Input: dimensioned drawing with shaded views. Units: mm. Origin: part minimum x, y, z. A direction names the side the tool comes from. Coordinates: 2 decimals unless noted, no trailing zeros. Order: outer loops, then holes, each group sorted by start corner. A loop starts at its lowest first (then second) coordinate and runs counter-clockwise, first axis right, second up. Notation, with made-up numbers: (71.25, 5.25) -> (112.25, 5.25) arc R22 cw to (112.25, 20.25) -> close; hole circle Ø11 at (72, 5.25). An arc over 180 degrees is marked (long way). Answer in a Markdown table with one row per item. Add a question column.
1) Pull-direction query (Z, two-part tool) for the marked faces 1, 2 and 3; classes: +Z half, -Z half, draft (parallel to the pull), parting line (faces both ways), or undercut.
2) Section query A-A on z = 0.4. Return the cut outline in (x, y), then the cut area to 3 significant figures.
3) Ray query, line 1 (Y direction, x = 20.82, z = 1.6); line 2 (X direction, y = 11, z = 1.75); line 3 (Y direction, x = 19.25, z = 2.75). Return the intervals inside material, ascending. Write a range as from..to.
4) Set-up query: the marked faces 4 and 5. Return all of +Z, -Z, +X, -X, +Y, -Y with unobstructed straight access to the full face (end or side cutting, diameter ignored); none if empty.
5) Section query C-C on y = 7.9. Return the cut outline in (x, z) (1 decimal).
6) Contact query for flat-ended pins moving along their axis: P1, Ø1, axis at x = 11, z = 1, coming from the -Y side; P2, Ø3.5, axis at x = 8.82, y = 34, coming from the +Z side (1 decimal). Output: stop coordinate, or through.
7) Section query D-D on y = 34. Return the cut outline in (x, z) (1 decimal).
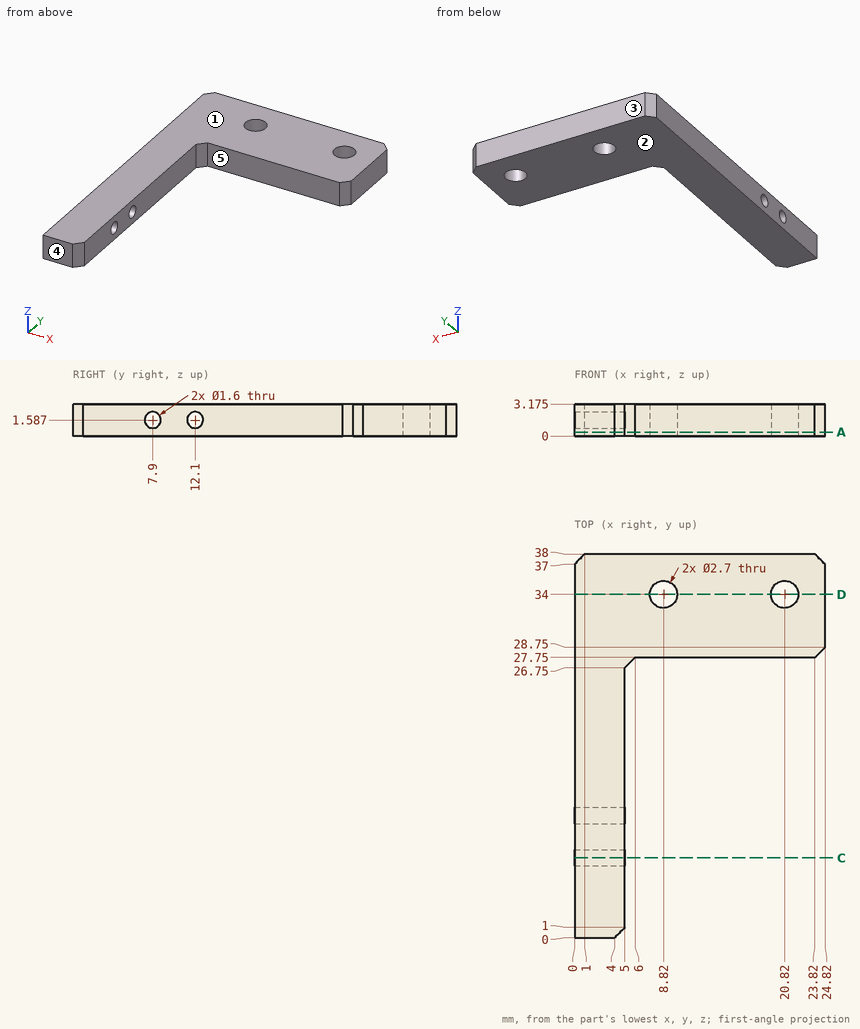
Result:
| question | item | result |
|---|---|---|
| 1 | face 1 | +Z half |
| 1 | face 2 | -Z half |
| 1 | face 3 | draft |
| 2 | outline | (0, 0) -> (4, 0) -> (5, 1) -> (5, 26.75) -> (6, 27.75) -> (23.82, 27.75) -> (24.82, 28.75) -> (24.82, 37) -> (23.82, 38) -> (1, 38) -> (0, 37) -> close; hole circle Ø2.7 at (8.82, 34); hole circle Ø2.7 at (20.82, 34) |
| 2 | area | 380 mm2 |
| 3 | line 1 | 27.75..32.65, 35.35..38 |
| 3 | line 2 | 0..5 |
| 3 | line 3 | 27.75..38 |
| 4 | face 4 | +Z, -Z, +X, -X, -Y |
| 4 | face 5 | +Z, -Z, +X, -Y |
| 5 | outline | (0, 0) -> (5, 0) -> (5, 0.8) -> (0, 0.8) -> close; (0, 2.4) -> (5, 2.4) -> (5, 3.2) -> (0, 3.2) -> close |
| 6 | P1 | y = 27.75 |
| 6 | P2 | z = 3.2 |
| 7 | outline | (0, 0) -> (7.5, 0) -> (7.5, 3.2) -> (0, 3.2) -> close; (10.2, 0) -> (19.5, 0) -> (19.5, 3.2) -> (10.2, 3.2) -> close; (22.2, 0) -> (24.8, 0) -> (24.8, 3.2) -> (22.2, 3.2) -> close |
